Solid Edge part; units mm, degrees
sketch "Sketch1" plane through (0, 0, 0) normal (0, 0, 1) x (1, 0, 0)
  line L0 (25, -25) -> (-25, -25)
  line L1 (-25, -25) -> (-25, 25)
  line L2 (-25, 25) -> (25, 25)
  line L3 (25, 25) -> (25, -25)
  dimension "D1" = 25
  dimension "D2" = 25
extrude "Protrusion1" add sketch "Sketch1" along normal blind 3
hole "Hole_1" at (-8, 8, 3) direction (0, 0, -1) diameter 2 end through all
hole "Hole1" at (-8, -8, 3) direction (0, 0, -1) diameter 2 end through all
hole "Hole2" at (8, -8, 3) direction (0, 0, -1) diameter 2 end through all
hole "Hole3" at (8, 8, 3) direction (0, 0, -1) diameter 2 end through all
hole "Hole_5" at (20, 20, 3) direction (0, 0, -1) diameter 3.2 end through all
hole "Hole4" at (20, -20, 3) direction (0, 0, -1) diameter 3.2 end through all
hole "Hole5" at (-20, -20, 3) direction (0, 0, -1) diameter 3.2 end through all
hole "Hole6" at (-20, 20, 3) direction (0, 0, -1) diameter 3.2 end through all
fillet "Round_1" radius 2 4 edges at (-25, -25, 1.5) (25, -25, 1.5) (-25, 25, 1.5) (25, 25, 1.5)
properties material "木材, アッシュ"
Could you check a few things on this model? Use its own coordinates, in mm. Give positions to 0.01 mm unless a question says otherwise; leave off trailing zeros. Write each loop counter-clockwise with the first axis right and the second up, starting at its lowest first coordinate (ties: lowest second). Pieces come first, ordered by that corner, then holes. Notation, with made-up numbers: (-33, 16) - (-25, 16) arc R28 cw to (-25, 46) - close; hole circle Ø4 at (57, 44). An arc over 180 degrees is marked (long way). One line per item, written item: value. Start each with the question number.
Item 1: Imagine slicing it at A-A, the plane y = 20. List the corners of the cut face in (x, z) for me, and give its area (3 significant figures).
Item 2: Please list where these lines run through material, in increasing order: line 1 (X direction, y = -8, z = 1.85); line 2 (X direction, y = 20, z = 2.1). Write a range as from..to.
Item 3: Imagine slicing it at C-C, the plane z = 1.4. Give the number of separate pieces and of enclosed holes in the cut face, and give its area (3 significant figures).
Item 4: Imagine slicing it at B-B, the plane x = 8. List the corners of the cut face in (y, z) for me.
Item 5: If we mould it in two halves opening along X, with no side actions, what happens to faces 1 (the face through (25, 0, 1)), 2 (the face through (-18.414, 20.208, 1.521)), 3 (the face through (0, 0, 3))? For each: +X half, -X half, draft (parallel to the pull), parting line (faces both ways), or undercut.
Item 6: I'm going to push a flat-ended pin straight in: pin 1 (3 mm diameter, centred on x = 20, y = 20, fed in from -Z). Where does the tip first touch, or does it pass through?
Geometry says:
1. outline: (-25, 0) - (-21.6, 0) - (-21.6, 3) - (-25, 3) - close; (-18.4, 0) - (18.4, 0) - (18.4, 3) - (-18.4, 3) - close; (21.6, 0) - (25, 0) - (25, 3) - (21.6, 3) - close
1. area: 131 mm^2
2. line 1: -25..-9, -7..7, 9..25
2. line 2: -25..-21.6, -18.4..18.4, 21.6..25
3. separate pieces: 1
3. enclosed holes: 8
3. area: 2,450 mm^2
4. outline: (-25, 0) - (-9, 0) - (-9, 3) - (-25, 3) - close; (-7, 0) - (7, 0) - (7, 3) - (-7, 3) - close; (9, 0) - (25, 0) - (25, 3) - (9, 3) - close
5. face 1: +X half
5. face 2: undercut
5. face 3: draft
6. pin 1: through
